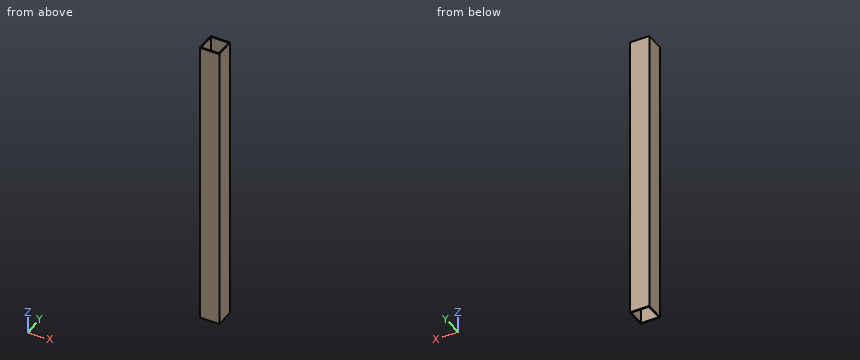
from build123d import *

# Parameters (mm, degrees)
SKETCH_1_W      = 20
SKETCH_1_H      = 20
SKETCH_1_W_2    = 18
SKETCH_1_H_2    = 18
EXTRUDE_1_DEPTH = 150
SKETCH_2_W      = 20
SKETCH_2_H      = 20
SKETCH_2_W_2    = 18
SKETCH_2_H_2    = 18
EXTRUDE_2_DEPTH = 150


with BuildPart() as part:
    # 草图1 → 凸台-拉伸1 (new body)
    with BuildSketch(Plane.XY):
        Rectangle(SKETCH_1_W, SKETCH_1_H)
        Rectangle(SKETCH_1_W_2, SKETCH_1_H_2, mode=Mode.SUBTRACT)
    extrude(amount=EXTRUDE_1_DEPTH)

    # 草图2 → 凸台-拉伸2 (add)
    with BuildSketch(Plane.XY.offset(150)):
        Rectangle(SKETCH_2_W, SKETCH_2_H)
        Rectangle(SKETCH_2_W_2, SKETCH_2_H_2, mode=Mode.SUBTRACT)
    extrude(amount=EXTRUDE_2_DEPTH)


solid = part.part
Input: part model. Units: mm. Frame: model coordinates. Give positions to 0.01 mm unless a question says otherwise; leave off trailing zeros. Order: outer loops, then holes, each group sorted by start corner. A loop starts at its lowest first (then second) coordinate and runs counter-clockwise, first axis right, second up.
Q1. Contact query for a flat-ended pin moving along its axis: pin 1 Ø3 at (x, y) = (3.5, -7) entering from -Z (3 decimals). Output: stop coordinate, or through.
Checked values:
pin 1: passes through
Q2. Ray query, probe 1 along Y at (x, z) = (-3.25, 137). Return the intervals inside material, ascending.
Checked values:
probe 1: y = -10 to -9, 9 to 10
Q3. Section B-B on z = 204.5. Output: boundary loops of the cut face in (x, y), and give its area (3 significant figures).
Checked values:
outline: (-10, -10) - (10, -10) - (10, 10) - (-10, 10) - close; hole (-9, -9) - (9, -9) - (9, 9) - (-9, 9) - close
area: 76.0 mm2
Q4. Section A-A on y = 2. Output: boundary loops of the cut face in (x, z), and give its area (3 significant figures).
Checked values:
outline: (-10, 0) - (-9, 0) - (-9, 300) - (-10, 300) - close; (9, 0) - (10, 0) - (10, 300) - (9, 300) - close
area: 600 mm2
